Part model, mm, in its own coordinate system. A direction names the side the tool comes from. Coordinates: 2 decimals unless noted, no trailing zeros. Order: outer loops, then holes, each group sorted by start corner. A loop starts at its lowest first (then second) coordinate and runs counter-clockwise, first axis right, second up.
1) Tool access for faces 4 (the flat face through (1, 0, 0)), 5 (the flat face through (1, 2.5, 0)): list every direction of +Z, -Z, +X, -X, +Y, -Y with a clear straight run to the whole face (end or side of a thin tool).
2) Pin check, flat tips, straight feed: pin 1 Ø3 at (x, z) = (1, 0.5) entering from -Y; pin 2 Ø1 at (y, z) = (1, -2) entering from -X; pin 3 Ø1.5 at (y, z) = (1.5, -0.5) entering from +X. Stop position of each tip, or through.
3) Mould opens along Z. For faces 1 (the cylindrical face through (-3.44, -0.35, 0.04)), 2 (the flat face through (-1, 0, -2.5)), 3 (the cylindrical face through (2.5, 1.2, 0)) say: +Z half, -Z half, draft (parallel to the pull), parting line (faces both ways), or undercut.
4) Cut at A-A (z = -0.4). List the corners of the cut face in (x, y), and give its area (3 significant figures).
5) Wall check: L1, parallel to Y at x = 0.25, z = -1.9; L2, parallel to X at y = -1, z = -0.15; L3, parallel to X at y = 1.75, z = -1.75. Give the ranges that are in metal, low to high.
6) Cut at D-D (z = -1.8). List the corners of the cut face in (x, y).
7) Cut at B-B (x = 2.25). List the corners of the cut face in (y, z).
8) Cut at C-C (y = -1.75). List the corners of the cut face in (x, z).
```python
from build123d import *

# Parameters (mm, degrees)
BOSS_EXTRUDE1_DEPTH = 2.5
SKETCH2_R           = 22
CUT_EXTRUDE1_DEPTH  = 9.383366498


with BuildPart() as part:
    # Sketch1 → Boss-Extrude1 (new, symmetric)
    with BuildSketch(Plane.XY):
        with BuildLine():
            Line((0, -2.732050808), (0, -3.291287847))
            ThreePointArc((0, -3.291287847), (-0.452277442, -4.127947874), (-1.4, -4.207802986))
            ThreePointArc((-1.4, -4.207802986), (-3.426172095, -0.284916247), (0, 2.5))
            Line((0, 2.5), (6.753938291, 2.5))
            Line((6.753938291, 2.5), (6.753938291, 0))
            Line((6.753938291, 0), (0, 0))
            ThreePointArc((0, 0), (-0.965925826, -0.741180955), (-0.5, -1.866025404))
            ThreePointArc((-0.5, -1.866025404), (-0.133974596, -2.232050808), (0, -2.732050808))
        make_face()
    extrude(amount=BOSS_EXTRUDE1_DEPTH, both=True)

    # Sketch2 → Cut-Extrude1 (cut, through all)
    with BuildSketch(Plane(origin=(0, 0, 0), x_dir=(1, 0, 0), z_dir=(0, 1, 0))):
        with Locations((24.5, 0)):
            Circle(SKETCH2_R)
    extrude(amount=CUT_EXTRUDE1_DEPTH, mode=Mode.SUBTRACT)


solid = part.part
```
Geometry check:
1. face 4: +Z, -Z, +X, -Y
1. face 5: +Z, -Z, +X, -X, +Y
2. pin 1: stops at y = -4.16
2. pin 2: stops at x = -3.16
2. pin 3: stops at x = 2.54
3. face 1: draft
3. face 2: -Z half
3. face 3: undercut
4. outline: (-1.4, -4.21) arc R1 ccw to (0, -3.29) - (0, -2.73) arc R1 ccw to (-0.5, -1.87) arc R1 cw to (0, 0) - (2.5, 0) - (2.5, 2.5) - (0, 2.5) arc R3.5 ccw to start
4. area: 23.5 mm2
5. L1: y = 0 to 2.5
5. L2: x = -3.5 to -1
5. L3: x = -2.17 to 2.57
6. outline: (-1.4, -4.21) arc R1 ccw to (0, -3.29) - (0, -2.73) arc R1 ccw to (-0.5, -1.87) arc R1 cw to (0, 0) - (2.57, 0) - (2.57, 2.5) - (0, 2.5) arc R3.5 ccw to start
7. outline: (0, -2.5) - (2.5, -2.5) - (2.5, 2.5) - (0, 2.5) - close
8. outline: (-3.42, -2.5) - (-0.66, -2.5) - (-0.66, 2.5) - (-3.42, 2.5) - close
